Design review of the part built by this model. Coordinates are the model's own, in mm. Give positions to 0.01 mm unless a question says otherwise; leave off trailing zeros. Write each loop counter-clockwise with the first axis right and the second up, starting at its lowest first coordinate (ties: lowest second). Pieces come first, ordered by that corner, then holes. Notation, with made-up numbers: (-14.75, 27) -> (4.25, 27) arc R22 cw to (4.25, 63) -> close; hole circle Ø3 at (20.5, 15). An arc over 180 degrees is marked (long way). Put each result on its own line as item: value. Start each with the question number.
from build123d import *

# Parameters (mm, degrees)
SKETCH2_W              = 50
SKETCH2_H              = 300
BOSS_EXTRUDE1_DEPTH    = 3.175
SKETCH3_R              = 1.025
SKETCH3_R_2            = 2.25
SKETCH3_W              = 29
SKETCH3_H              = 60
SKETCH3_W_2            = 28.48
SKETCH3_H_2            = 59.03
CUT_EXTRUDE1_DEPTH     = 6.35
CUT_EXTRUDE2_DEPTH     = 6.35
SKETCH5_R              = 3.175
SKETCH5_W              = 20
SKETCH5_H              = 70
CUT_EXTRUDE3_DEPTH     = 6.35
M2_5_CLEARANCE_HOLE1_D = 2.9


with BuildPart() as part:
    # Sketch2 → Boss-Extrude1 (new body)
    with BuildSketch(Plane(origin=(0, 0, 0), x_dir=(1, 0, 0), z_dir=(0, 1, 0))):
        with Locations((25, -150)):
            Rectangle(SKETCH2_W, SKETCH2_H)
    extrude(amount=BOSS_EXTRUDE1_DEPTH)

    # Sketch3 → Cut-Extrude1 (cut)
    with BuildSketch(Plane(origin=(0, 3.175, 0), x_dir=(1, 0, 0), z_dir=(0, 1, 0))):
        with Locations(Location((7.7, -21, 0), (0, 0, 270))):
            Circle(SKETCH3_R)
        with Locations(Location((7.7, -43, 0), (0, 0, 270))):
            Circle(SKETCH3_R)
        with Locations(Location((7.7, -65, 0), (0, 0, 270))):
            Circle(SKETCH3_R)
        with Locations(Location((42.3, -65, 0), (0, 0, 270))):
            Circle(SKETCH3_R)
        with Locations(Location((42.3, -43, 0), (0, 0, 270))):
            Circle(SKETCH3_R)
        with Locations(Location((42.3, -21, 0), (0, 0, 270))):
            Circle(SKETCH3_R)
        with Locations(Location((16.5, -292.24, 0), (0, 0, 270))):
            Circle(SKETCH3_R_2)
        with Locations(Location((33.5, -292.24, 0), (0, 0, 270))):
            Circle(SKETCH3_R_2)
        with Locations(Location((16.5, -222.41, 0), (0, 0, 270))):
            Circle(SKETCH3_R_2)
        with Locations(Location((33.5, -222.41, 0), (0, 0, 270))):
            Circle(SKETCH3_R_2)
        with Locations((25, -40.5)):
            Rectangle(SKETCH3_W, SKETCH3_H)
        with Locations((25, -257.325)):
            Rectangle(SKETCH3_W_2, SKETCH3_H_2)
    extrude(amount=-CUT_EXTRUDE1_DEPTH, mode=Mode.SUBTRACT)

    # Sketch4 → Cut-Extrude2 (cut)
    with BuildSketch(Plane(origin=(0, 3.175, 0), x_dir=(1, 0, 0), z_dir=(0, 1, 0))):
        with BuildLine():
            Line((0, 0), (0, -25))
            ThreePointArc((0, -25), (7.32233047, -7.32233047), (25, 0))
            Line((25, 0), (0, 0))
        make_face()
        with BuildLine():
            ThreePointArc((25, 0), (42.67766953, -7.32233047), (50, -25))
            Line((50, -25), (50, 0))
            Line((50, 0), (25, 0))
        make_face()
        with BuildLine():
            ThreePointArc((25, -300), (7.32233047, -292.67766953), (0, -275))
            Line((0, -275), (0, -300))
            Line((0, -300), (25, -300))
        make_face()
        with BuildLine():
            Line((50, -300), (50, -275))
            ThreePointArc((50, -275), (42.67766953, -292.67766953), (25, -300))
            Line((25, -300), (50, -300))
        make_face()
    extrude(amount=-CUT_EXTRUDE2_DEPTH, mode=Mode.SUBTRACT)

    # Sketch5 → Cut-Extrude3 (cut)
    with BuildSketch(Plane.XZ):
        with Locations(Location((12.5, 205, 0), (0, 0, 270))):
            Circle(SKETCH5_R)
        with Locations(Location((12.5, 95, 0), (0, 0, 90))):
            Circle(SKETCH5_R)
        with Locations(Location((37.5, 95, 0), (0, 0, 270))):
            Circle(SKETCH5_R)
        with Locations(Location((37.5, 205, 0), (0, 0, 90))):
            Circle(SKETCH5_R)
        with Locations((25, 150)):
            Rectangle(SKETCH5_W, SKETCH5_H)
    extrude(amount=-CUT_EXTRUDE3_DEPTH, mode=Mode.SUBTRACT)

    # M2.5 Clearance Hole1 (through all)
    with Locations(Plane(origin=(0, 0, 0), x_dir=(-1, 0, 0), z_dir=(0, -1, 0))):
        with Locations((-7.7, -65), (-42.3, -65), (-7.7, -43), (-42.3, -43), (-42.3, -21), (-7.7, -21)):
            Hole(M2_5_CLEARANCE_HOLE1_D / 2)


solid = part.part
Q1. Take a section at A-A on z = 243.5. Give the boundary of the cut face in (x, y) (3 decimals).
Q2. Take a section at B-B on y = 0.5. State how many separate pieces and enclosed holes the cut face has, then the cut area to 3 significant figures.
Q3. To check wall thickness, follow probe 1 along X at (y, z) = (1.5, 95) (3 decimals); probe 2 along X at (y, z) = (1.15, 43); probe 3 along Z at (x, y) = (24.5, 1.95) (3 decimals). State the ranges of each line that lie inside material, in increasing order. Write a range as from..to.
Q4. For pin 1 (1.6 mm diameter, centred on x = 23.5, y = 2, fed in from +Z), flat-tipped, find the tip position at first contact; note if it passes through.
Q5. Mouldability with a two-part tool opening along Z and no side actions: class faces 1 (the face through (37.36, 1.57, 201.83)), 2 (the face through (36, 0, 148)) as +Z half, -Z half, draft (parallel to the pull), parting line (faces both ways), or undercut.
Result:
1. outline: (0, 0) -> (10.76, 0) -> (10.76, 3.175) -> (0, 3.175) -> close; (39.24, 0) -> (50, 0) -> (50, 3.175) -> (39.24, 3.175) -> close
2. separate pieces: 1
2. enclosed holes: 17
2. area: 9,410 mm^2
3. probe 1: x = 0..9.325, 15.675..34.325, 40.675..50
3. probe 2: x = 0..6.25, 9.15..10.5, 39.5..40.85, 43.75..50
3. probe 3: z = 0.005..10.5, 70.5..115, 185..227.81, 286.84..299.995
4. pin 1: stops at z = 299.99
5. face 1: undercut
5. face 2: draft
